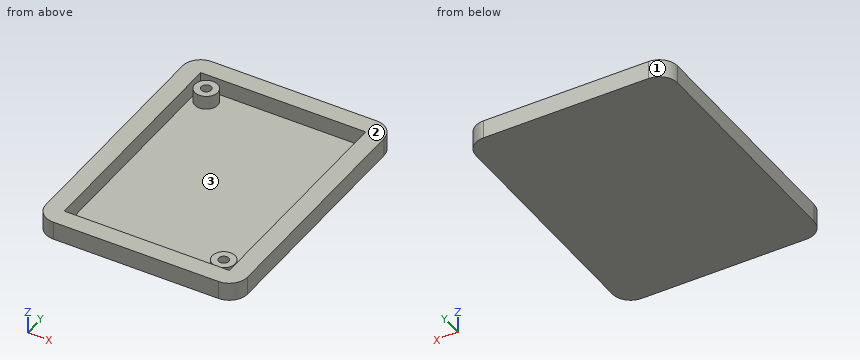
```python
from build123d import *

# Parameters (mm, degrees)
SKETCH_W      = 44
SKETCH_H      = 58
PAD_DEPTH     = 4
SKETCH001_W   = 36
SKETCH001_H   = 50
POCKET_DEPTH  = 3.6
SKETCH002_R   = 2.5
SKETCH002_R_2 = 1.1
PAD001_DEPTH  = 3
FILLET_R      = 4


with BuildPart() as part:
    # Sketch → Pad (new body)
    with BuildSketch(Plane.XY):
        Rectangle(SKETCH_W, SKETCH_H)
    extrude(amount=PAD_DEPTH)

    # Sketch001 (on Face6 of Pad) → Pocket (cut)
    with BuildSketch(Plane.XY.offset(4)):
        Rectangle(SKETCH001_W, SKETCH001_H)
    extrude(amount=-POCKET_DEPTH, mode=Mode.SUBTRACT)

    # Sketch002 (on Face11 of Pocket) → Pad001 (join)
    with BuildSketch(Plane.XY.offset(0.4)):
        with Locations((-15, 22)):
            Circle(SKETCH002_R)
        with Locations((-15, 22)):
            Circle(SKETCH002_R_2, mode=Mode.SUBTRACT)
        with Locations((15, -22)):
            Circle(SKETCH002_R)
        with Locations((15, -22)):
            Circle(SKETCH002_R_2, mode=Mode.SUBTRACT)
    extrude(amount=PAD001_DEPTH)

    # Fillet
    fillet_edges = [part.edges().sort_by_distance(p)[0] for p in [
        (-22, -29, 2),
        (22, -29, 2),
        (22, 29, 2),
        (-22, 29, 2),
    ]]
    fillet(fillet_edges, radius=FILLET_R)


solid = part.part
```
CAD build for the part. Positions are in the model's coordinates, mm. Face numbers are marked on the shaded views. Give positions to 0.01 mm unless a question says otherwise; leave off trailing zeros. Write each loop counter-clockwise with the first axis right and the second up, starting at its lowest first coordinate (ties: lowest second). Pieces come first, ordered by that corner, then holes. Notation, with made-up numbers: M 81,68 L 113,68 A26 cw 113,96 Z; hole C 58,-12 d7. An arc over 180 degrees is marked long. Return JSON: item names as keys, results as strings. Group by question number.
(1) Flat gauge pins, fed straight in: pin 1 Ø2.5 at (x, y) = (-16, 21) entering from +Z; pin 2 Ø2 at (x, y) = (-15, 22) entering from +Z; pin 3 Ø5.5 at (x, y) = (16, -22) entering from +Z. Where does each tip first touch, or does it go through?
(2) Band-saw the part on C-C (y = 22). Give the cut face in (x, z).
(3) Band-saw the part on A-A (z = 2.3). Give the cut face in (x, y), and give its area (3 significant figures).
(4) Mould opens along X. For the marked faces 1, 2 and 3 say: pulls with the +X half, pulls with the -X half, needs draft (parallel to the pull), parting line crosses it, or undercut.
(5) Band-saw the part on D-D (x = -15). Give the cut face in (y, z).
(6) Band-saw the part on B-B (x = -4). Give the cut face in (y, z), and give its area (3 significant figures).
(7) Drill centre lines: L1, parallel to Y at x = -15, z = 2.4; L2, parallel to X at y = -3, z = 2.1; L3, parallel to Y at x = 15, z = 2.15. Where is each one in solid material? Low to high. Write a range as [from, to].
Entries:
{
 "1": {"pin 1": "stops at z = 3.4", "pin 2": "stops at z = 0.4", "pin 3": "stops at z = 4"},
 "2": {"outline": "M -22,0 L 22,0 L 22,4 L 18,4 L 18,0.4 L -12.5,0.4 L -12.5,3.4 L -13.9,3.4 L -13.9,0.4 L -16.1,0.4 L -16.1,3.4 L -17.5,3.4 L -17.5,0.4 L -18,0.4 L -18,4 L -22,4 Z"},
 "3": {"outline": "M -22,-25 A4 ccw -18,-29 L 18,-29 A4 ccw 22,-25 L 22,25 A4 ccw 18,29 L -18,29 A4 ccw -22,25 Z; C -15,22 d5; C 15,-22 d5; hole M -18,-25 L 18,-25 L 18,25 L -18,25 Z; hole C -15,22 d2.2; hole C 15,-22 d2.2", "area": "770 mm^2"},
 "4": {"face 1": "pulls with the -X half", "face 2": "needs draft", "face 3": "undercut"},
 "5": {"outline": "M -29,0 L 29,0 L 29,4 L 25,4 L 25,0.4 L 24.5,0.4 L 24.5,3.4 L 23.1,3.4 L 23.1,0.4 L 20.9,0.4 L 20.9,3.4 L 19.5,3.4 L 19.5,0.4 L -25,0.4 L -25,4 L -29,4 Z"},
 "6": {"outline": "M -29,0 L 29,0 L 29,4 L 25,4 L 25,0.4 L -25,0.4 L -25,4 L -29,4 Z", "area": "52.0 mm^2"},
 "7": {"L1": "y = [-29, -25], [19.5, 20.9], [23.1, 24.5], [25, 29]", "L2": "x = [-22, -18], [18, 22]", "L3": "y = [-29, -25], [-24.5, -23.1], [-20.9, -19.5], [25, 29]"}
}
